```python
from build123d import *

# Parameters (mm, degrees)
SKETCH1_W             = 23
SKETCH1_H             = 21
EXTRUDE1_DEPTH        = 5
SKETCH2_R             = 2.15
EXTRUDE2_DEPTH        = 4.5
SKETCH4_R             = 1.25
EXTRUDE4_DEPTH        = 8
FILLET1_R             = 5
SKETCH6_R             = 2.05
EXTRUDE6_DEPTH        = 4.5
SKETCH9_W             = 12
SKETCH9_H             = 26
EXTRUDE9_DEPTH        = 5
SKETCH11_R            = 1.7
EXTRUDE11_DEPTH       = 5
SKETCH10_R            = 2
EXTRUDE10_DEPTH       = 4
M3_TAPPED_HOLE1_D     = 2.5
M3_TAPPED_HOLE1_DEPTH = 8
M3_TAPPED_HOLE1_TIP   = 0.751075774
FILLET3_R             = 3
EXTRUDE15_DEPTH       = 5
FILLET6_R             = 2
SKETCH16_R            = 0.75
EXTRUDE16_DEPTH       = 5
M3_TAPPED_HOLE2_D     = 2.5
M3_TAPPED_HOLE2_DEPTH = 7.5
M3_TAPPED_HOLE2_TIP   = 0.751075774


with BuildPart() as part:
    # Sketch1 → Extrude1 (new body)
    with BuildSketch(Plane.XY):
        with Locations((3.5, -4)):
            Rectangle(SKETCH1_W, SKETCH1_H)
    extrude(amount=EXTRUDE1_DEPTH)

    # Sketch2 → Extrude2 (cut)
    with BuildSketch(Plane.XY.offset(5)):
        with Locations((6, 0)):
            Circle(SKETCH2_R)
    extrude(amount=-EXTRUDE2_DEPTH, mode=Mode.SUBTRACT)

    # Sketch4 → Extrude4 (cut)
    with BuildSketch(Plane.XZ.offset(14.5)):
        with Locations(Location((-1.4, 2.5, 0), (0, 0, 270))):
            Circle(SKETCH4_R)
        with Locations(Location((12, 2.5, 0), (0, 0, 270))):
            Circle(SKETCH4_R)
    extrude(amount=-EXTRUDE4_DEPTH, mode=Mode.SUBTRACT)

    # Fillet1
    fillet1_edges = [part.edges().sort_by_distance(p)[0] for p in [
        (15, 6.5, 2.5),
    ]]
    fillet(fillet1_edges, radius=FILLET1_R)

    # Sketch6 → Extrude6 (cut)
    with BuildSketch(Plane(origin=(0, 0, 0), x_dir=(-1, 0, 0), z_dir=(0, 0, -1))):
        with Locations((-4.9, -6.5)):
            Circle(SKETCH6_R)
    extrude(amount=-EXTRUDE6_DEPTH, mode=Mode.SUBTRACT)

    # Sketch9 → Extrude9 (add)
    with BuildSketch(Plane(origin=(0, 0, 0), x_dir=(-1, 0, 0), z_dir=(0, 0, -1))):
        with Locations((14, -6.5)):
            Rectangle(SKETCH9_W, SKETCH9_H)
    extrude(amount=-EXTRUDE9_DEPTH)

    # Sketch11 → Extrude11 (cut)
    with BuildSketch(Plane.XY.offset(5)):
        with Locations((-17.5, -5.5)):
            Circle(SKETCH11_R)
    extrude(amount=-EXTRUDE11_DEPTH, mode=Mode.SUBTRACT)

    # Sketch10 → Extrude10 (cut)
    with BuildSketch(Plane.XY.offset(5)):
        with Locations((-10, -2.5)):
            Circle(SKETCH10_R)
    extrude(amount=-EXTRUDE10_DEPTH, mode=Mode.SUBTRACT)

    # M3 Tapped Hole1
    with Locations(Plane(origin=(-1.4, -14.5, 2.5), x_dir=(0, 0, -1), z_dir=(0, -1, 0))):
        with Locations((0, 0), (0, 13.4)):
            Hole(M3_TAPPED_HOLE1_D / 2, depth=M3_TAPPED_HOLE1_DEPTH)
            with Locations((0, 0, -(M3_TAPPED_HOLE1_DEPTH + M3_TAPPED_HOLE1_TIP / 2))):  # 118° drill point
                Cone(0, M3_TAPPED_HOLE1_D / 2, M3_TAPPED_HOLE1_TIP, mode=Mode.SUBTRACT)

    # Fillet3
    fillet3_edges = [part.edges().sort_by_distance(p)[0] for p in [
        (-20, -19.5, 2.5),
        (-20, 6.5, 2.5),
    ]]
    fillet(fillet3_edges, radius=FILLET3_R)

    # Sketch15 → Extrude15 (cut)
    with BuildSketch(Plane.XY.offset(5)):
        Polygon((-14, 2.5), (-17, 6.5), (-7, 6.5), (-10, 2.5), align=None)
    extrude(amount=-EXTRUDE15_DEPTH, mode=Mode.SUBTRACT)

    # Fillet6
    fillet6_edges = [part.edges().sort_by_distance(p)[0] for p in [
        (-10, 2.5, 2.5),
        (-14, 2.5, 2.5),
    ]]
    fillet(fillet6_edges, radius=FILLET6_R)

    # Sketch16 → Extrude16 (cut)
    with BuildSketch(Plane(origin=(0, 0, 0), x_dir=(-1, 0, 0), z_dir=(0, 0, -1))):
        with Locations((17, -11)):
            Circle(SKETCH16_R)
        with Locations((8, -11)):
            Circle(SKETCH16_R)
    extrude(amount=-EXTRUDE16_DEPTH, mode=Mode.SUBTRACT)

    # M3 Tapped Hole2
    with Locations(Plane(origin=(-8, -11, 0), x_dir=(-1, 0, 0), z_dir=(0, 0, -1))):
        with Locations((0, 0), (9, 0)):
            Hole(M3_TAPPED_HOLE2_D / 2, depth=M3_TAPPED_HOLE2_DEPTH)
            with Locations((0, 0, -(M3_TAPPED_HOLE2_DEPTH + M3_TAPPED_HOLE2_TIP / 2))):  # 118° drill point
                Cone(0, M3_TAPPED_HOLE2_D / 2, M3_TAPPED_HOLE2_TIP, mode=Mode.SUBTRACT)


solid = part.part
```
Geometry check sheet. Reference: the model listing, model coordinates, mm. A direction names the side the tool comes from. Round coordinates to 2 decimals unless told otherwise and drop trailing zeros. Loops run counter-clockwise (first coordinate to the right, second up) from the corner with the lowest first, then second, coordinate; pieces in that order, holes last. Notation, with made-up numbers: (-39, 23.5) -> (14, 23.5) arc R19 cw to (14, 33.5) -> close; hole circle Ø4 at (23, -23). An arc over 180 degrees is marked (long way). Use a Markdown table: item, result.
(1) Scan lines: probe 1 along X at (y, z) = (-13, 2.55); probe 2 along Y at (x, z) = (-17.5, 1.6); probe 3 along X at (y, z) = (-4.25, 1.5). Record each from-to range of solid material in increasing order.
Calculated:
| item | result |
|---|---|
| probe 1 | -20 to -2.65, -0.15 to 10.75, 13.25 to 15 |
| probe 2 | -19.46 to -12.15, -9.85 to -7.2, -3.8 to 6.46 |
| probe 3 | -20 to -18.65, -16.35 to -10.97, -9.03 to 15 |
(2) Set-up check for faces 4 (the flat face through (-8.2, 4.9, 2.5)), 5 (the cylindrical face through (13.054, -10.556, 1.828)), 6 (the flat face through (3, -14.5, 2)): record each of +Z, -Z, +X, -X, +Y, -Y from which the full face is reachable in a straight line by a thin tool's end or side.
Calculated:
| item | result |
|---|---|
| face 4 | +Z, -Z, +Y |
| face 5 | -Y |
| face 6 | +Z, -Z, +X, -Y |
(3) Sectioned sample at B-B (x = -16.5). Enter the section's corners in (y, z).
Calculated:
| item | result |
|---|---|
| outline | (-19.5, 0) -> (-12.15, 0) -> (-12.15, 5) -> (-19.5, 5) -> close; (-9.85, 0) -> (-6.87, 0) -> (-6.87, 5) -> (-9.85, 5) -> close; (-4.13, 0) -> (5.83, 0) -> (5.83, 5) -> (-4.13, 5) -> close |
(4) Sectioned sample at A-A (y = 0). Enter the section's corners in (x, z).
Calculated:
| item | result |
|---|---|
| outline | (-20, 0) -> (15, 0) -> (15, 5) -> (8.15, 5) -> (8.15, 0.5) -> (3.85, 0.5) -> (3.85, 5) -> (-20, 5) -> close |
(5) Go/stop test with flat-tipped pins: P1, Ø3, axis at x = -1.4, z = 2.5, coming from the -Y side; P2, Ø5, axis at x = -10, y = -2.5, coming from the +Z side; P3, Ø4, axis at x = 6, y = 0, coming from the +Z side; P4, Ø0.6, axis at x = -12.5, z = 1.5, coming from the +Y side. Record where each tip stops, or that it passes through.
Calculated:
| item | result |
|---|---|
| P1 | y = -14.5 |
| P2 | z = 5 |
| P3 | z = 0.5 |
| P4 | y = 2.5 |
(6) Sectioned sample at C-C (x = 6). Enter the section's corners in (y, z), then the cut area to 3 significant figures.
Calculated:
| item | result |
|---|---|
| outline | (-14.5, 0) -> (-8.23, 0) -> (-8.23, 4.5) -> (-4.77, 4.5) -> (-4.77, 0) -> (6.5, 0) -> (6.5, 5) -> (2.15, 5) -> (2.15, 0.5) -> (-2.15, 0.5) -> (-2.15, 5) -> (-14.5, 5) -> close |
| area | 70.1 mm² |
(7) Mould release check, pull along X, two halves, no side actions. Record for faces 1 (the cylindrical face through (-15.93, -6.15, 2.54)), 2 (the cylindrical face through (13.5, 5.07, 2.54)), 3 (the flat face through (-20, -7, 2)): released by +X, released by -X, zero draft, split by the parting line, or undercut.
Calculated:
| item | result |
|---|---|
| face 1 | undercut |
| face 2 | released by +X |
| face 3 | released by -X |
(8) Sectioned sample at D-D (x = -6). Enter the section's corners in (y, z), then the cut area to 3 significant figures.
Calculated:
| item | result |
|---|---|
| outline | (-14.5, 0) -> (6.5, 0) -> (6.5, 5) -> (-14.5, 5) -> close |
| area | 105 mm² |
